from build123d import *

# Parameters (mm, degrees)
BOSS_EXTRUDE1_DEPTH = 100.5


with BuildPart() as part:
    # Sketch1 → Boss-Extrude1 (new body)
    with BuildSketch(Plane(origin=(0, 0, 0), x_dir=(0, 0, -1), z_dir=(1, 0, 0))):
        with BuildLine():
            Line((-15, 13), (-15, 4))
            Line((-15, 4), (-13, 4))
            Line((-13, 4), (-13, 8.25))
            Line((-13, 8.25), (-9.664213562, 8.25))
            Line((-9.664213562, 8.25), (-6, 4.585786438))
            Line((-6, 4.585786438), (-6, -4.585786438))
            Line((-6, -4.585786438), (-9.664213562, -8.25))
            Line((-9.664213562, -8.25), (-13, -8.25))
            Line((-13, -8.25), (-13, -4))
            Line((-13, -4), (-15, -4))
            Line((-15, -4), (-15, -13))
            ThreePointArc((-15, -13), (-14.414213562, -14.414213562), (-13, -15))
            Line((-13, -15), (-4, -15))
            Line((-4, -15), (-4, -13))
            Line((-4, -13), (-8.25, -13))
            Line((-8.25, -13), (-8.25, -9.664213562))
            Line((-8.25, -9.664213562), (-4.585786438, -6))
            Line((-4.585786438, -6), (4.585786438, -6))
            Line((4.585786438, -6), (8.25, -9.664213562))
            Line((8.25, -9.664213562), (8.25, -13))
            Line((8.25, -13), (4, -13))
            Line((4, -13), (4, -15))
            Line((4, -15), (13, -15))
            ThreePointArc((13, -15), (14.414213562, -14.414213562), (15, -13))
            Line((15, -13), (15, -4))
            Line((15, -4), (13, -4))
            Line((13, -4), (13, -8.25))
            Line((13, -8.25), (9.664213562, -8.25))
            Line((9.664213562, -8.25), (6, -4.585786438))
            Line((6, -4.585786438), (6, 4.585786438))
            Line((6, 4.585786438), (9.664213562, 8.25))
            Line((9.664213562, 8.25), (13, 8.25))
            Line((13, 8.25), (13, 4))
            Line((13, 4), (15, 4))
            Line((15, 4), (15, 13))
            ThreePointArc((15, 13), (14.414213562, 14.414213562), (13, 15))
            Line((13, 15), (4, 15))
            Line((4, 15), (4, 13))
            Line((4, 13), (8.25, 13))
            Line((8.25, 13), (8.25, 9.664213562))
            Line((8.25, 9.664213562), (4.585786438, 6))
            Line((4.585786438, 6), (-4.585786438, 6))
            Line((-4.585786438, 6), (-8.25, 9.664213562))
            Line((-8.25, 9.664213562), (-8.25, 13))
            Line((-8.25, 13), (-4, 13))
            Line((-4, 13), (-4, 15))
            Line((-4, 15), (-13, 15))
            ThreePointArc((-13, 15), (-14.414213562, 14.414213562), (-15, 13))
        make_face()
        with BuildLine():
            Line((-9.539070071, 11.338915743), (-9.918883282, 12.361530981))
            ThreePointArc((-9.918883282, 12.361530981), (-13.043502884, 13.043502884), (-12.361530981, 9.918883282))
            Line((-12.361530981, 9.918883282), (-11.338915743, 9.539070071))
            ThreePointArc((-11.338915743, 9.539070071), (-9.861522369, 9.861522369), (-9.539070071, 11.338915743))
        make_face(mode=Mode.SUBTRACT)
        with BuildLine():
            Line((9.918883282, 12.361530981), (9.539070071, 11.338915743))
            ThreePointArc((9.539070071, 11.338915743), (9.861522369, 9.861522369), (11.338915743, 9.539070071))
            Line((11.338915743, 9.539070071), (12.361530981, 9.918883282))
            ThreePointArc((12.361530981, 9.918883282), (13.043502884, 13.043502884), (9.918883282, 12.361530981))
        make_face(mode=Mode.SUBTRACT)
        with BuildLine():
            Line((12.361530981, -9.918883282), (11.338915743, -9.539070071))
            ThreePointArc((11.338915743, -9.539070071), (9.861522369, -9.861522369), (9.539070071, -11.338915743))
            Line((9.539070071, -11.338915743), (9.918883282, -12.361530981))
            ThreePointArc((9.918883282, -12.361530981), (13.043502884, -13.043502884), (12.361530981, -9.918883282))
        make_face(mode=Mode.SUBTRACT)
        with BuildLine():
            Line((-11.338915743, -9.539070071), (-12.361530981, -9.918883282))
            ThreePointArc((-12.361530981, -9.918883282), (-13.043502884, -13.043502884), (-9.918883282, -12.361530981))
            Line((-9.918883282, -12.361530981), (-9.539070071, -11.338915743))
            ThreePointArc((-9.539070071, -11.338915743), (-9.861522369, -9.861522369), (-11.338915743, -9.539070071))
        make_face(mode=Mode.SUBTRACT)
        with BuildLine():
            Line((-4.8, -2.644433572), (-4.8, -4.5))
            ThreePointArc((-4.8, -4.5), (-4.712132034, -4.712132034), (-4.5, -4.8))
            Line((-4.5, -4.8), (-2.644433572, -4.8))
            ThreePointArc((-2.644433572, -4.8), (-2.615679847, -4.79861886), (-2.587190874, -4.794488155))
            Line((-2.587190874, -4.794488155), (-1.742757301, -4.630346896))
            ThreePointArc((-1.742757301, -4.630346896), (-1.568512625, -4.526682207), (-1.5, -4.335858741))
            Line((-1.5, -4.335858741), (-1.5, -3.5))
            ThreePointArc((-1.5, -3.5), (-1.374371458, -3.255879959), (-1.102702703, -3.216216216))
            ThreePointArc((-1.102702703, -3.216216216), (0, -3.4), (1.102702703, -3.216216216))
            ThreePointArc((1.102702703, -3.216216216), (1.374371458, -3.255879959), (1.5, -3.5))
            Line((1.5, -3.5), (1.5, -4.335858741))
            ThreePointArc((1.5, -4.335858741), (1.568512625, -4.526682207), (1.742757301, -4.630346896))
            Line((1.742757301, -4.630346896), (2.587190874, -4.794488155))
            ThreePointArc((2.587190874, -4.794488155), (2.615679847, -4.79861886), (2.644433572, -4.8))
            Line((2.644433572, -4.8), (4.5, -4.8))
            ThreePointArc((4.5, -4.8), (4.712132034, -4.712132034), (4.8, -4.5))
            Line((4.8, -4.5), (4.8, -2.644433572))
            ThreePointArc((4.8, -2.644433572), (4.79861886, -2.615679847), (4.794488155, -2.587190874))
            Line((4.794488155, -2.587190874), (4.630346896, -1.742757301))
            ThreePointArc((4.630346896, -1.742757301), (4.526682207, -1.568512625), (4.335858741, -1.5))
            Line((4.335858741, -1.5), (3.5, -1.5))
            ThreePointArc((3.5, -1.5), (3.255879959, -1.374371458), (3.216216216, -1.102702703))
            ThreePointArc((3.216216216, -1.102702703), (3.4, 0), (3.216216216, 1.102702703))
            ThreePointArc((3.216216216, 1.102702703), (3.255879959, 1.374371458), (3.5, 1.5))
            Line((3.5, 1.5), (4.335858741, 1.5))
            ThreePointArc((4.335858741, 1.5), (4.526682207, 1.568512625), (4.630346896, 1.742757301))
            Line((4.630346896, 1.742757301), (4.794488155, 2.587190874))
            ThreePointArc((4.794488155, 2.587190874), (4.79861886, 2.615679847), (4.8, 2.644433572))
            Line((4.8, 2.644433572), (4.8, 4.5))
            ThreePointArc((4.8, 4.5), (4.712132034, 4.712132034), (4.5, 4.8))
            Line((4.5, 4.8), (2.644433572, 4.8))
            ThreePointArc((2.644433572, 4.8), (2.615679847, 4.79861886), (2.587190874, 4.794488155))
            Line((2.587190874, 4.794488155), (1.742757301, 4.630346896))
            ThreePointArc((1.742757301, 4.630346896), (1.568512625, 4.526682207), (1.5, 4.335858741))
            Line((1.5, 4.335858741), (1.5, 3.5))
            ThreePointArc((1.5, 3.5), (1.374371458, 3.255879959), (1.102702703, 3.216216216))
            ThreePointArc((1.102702703, 3.216216216), (0, 3.4), (-1.102702703, 3.216216216))
            ThreePointArc((-1.102702703, 3.216216216), (-1.374371458, 3.255879959), (-1.5, 3.5))
            Line((-1.5, 3.5), (-1.5, 4.335858741))
            ThreePointArc((-1.5, 4.335858741), (-1.568512625, 4.526682207), (-1.742757301, 4.630346896))
            Line((-1.742757301, 4.630346896), (-2.587190874, 4.794488155))
            ThreePointArc((-2.587190874, 4.794488155), (-2.615679847, 4.79861886), (-2.644433572, 4.8))
            Line((-2.644433572, 4.8), (-4.5, 4.8))
            ThreePointArc((-4.5, 4.8), (-4.712132034, 4.712132034), (-4.8, 4.5))
            Line((-4.8, 4.5), (-4.8, 2.644433572))
            ThreePointArc((-4.8, 2.644433572), (-4.79861886, 2.615679847), (-4.794488155, 2.587190874))
            Line((-4.794488155, 2.587190874), (-4.630346896, 1.742757301))
            ThreePointArc((-4.630346896, 1.742757301), (-4.526682207, 1.568512625), (-4.335858741, 1.5))
            Line((-4.335858741, 1.5), (-3.5, 1.5))
            ThreePointArc((-3.5, 1.5), (-3.255879959, 1.374371458), (-3.216216216, 1.102702703))
            ThreePointArc((-3.216216216, 1.102702703), (-3.4, 0), (-3.216216216, -1.102702703))
            ThreePointArc((-3.216216216, -1.102702703), (-3.255879959, -1.374371458), (-3.5, -1.5))
            Line((-3.5, -1.5), (-4.335858741, -1.5))
            ThreePointArc((-4.335858741, -1.5), (-4.526682207, -1.568512625), (-4.630346896, -1.742757301))
            Line((-4.630346896, -1.742757301), (-4.794488155, -2.587190874))
            ThreePointArc((-4.794488155, -2.587190874), (-4.79861886, -2.615679847), (-4.8, -2.644433572))
        make_face(mode=Mode.SUBTRACT)
    extrude(amount=BOSS_EXTRUDE1_DEPTH)


solid = part.part
Source: CAD feature listing. Evaluate the final solid. Frame: model axes, mm. A direction names the side the tool comes from. Give positions to 0.01 mm unless a question says otherwise; leave off trailing zeros. Write item = value, one per line.
Q1. First-contact query: pin 1 (0.6 mm diameter, centred on x = 74.5, y = 14.5, fed in from -Z); pin 2 (2 mm diameter, centred on y = 7, z = 6, fed in from -X). Flat tips, straight axial feed; report the tip coordinate or a pass-through.
Here are the results:
pin_1 = -14.6
pin_2 = 0
Q2. Cut plane A-A on x = 23. State how many separate pieces and enclosed holes the cut face has, then the cut area to 3 significant figures.
Here are the results:
separate_pieces = 1
enclosed_holes = 5
area = 299 mm²
Q3. Reachability of faces 4 (the face through (50, 6, -13)), 5 (the face through (50, 14, -4)), 6 (the face through (50, 8, -15)) from +Z, -Z, +X, -X, +Y, -Y: full face, straight path, thin tool, end or side. Return the list, or none.
Here are the results:
face_4 = +X, -X
face_5 = +X, -X, +Y
face_6 = -Z, +X, -X, +Y, -Y
Q4. Line query: line 1 (Y direction, x = 50.5, z = -11.7); line 2 (Z direction, x = 19, y = 12.75). Output: solid intervals per line, ascending. Write a range as from..to.
Here are the results:
line_1 = -15..-13.6, -9.67..-8.25, 8.25..9.67, 13.6..15
line_2 = -15..-13.28, -10.12..-8.25, 8.25..10.12, 13.28..15
Q5. Mould query, pull axis Z, two halves, no side actions, for faces 1 (the face through (50, 15, 8)), 2 (the face through (50, -9, -15)), 3 (the face through (49.546, -9.877, 9.846)). Classes: +Z half, -Z half, draft (parallel to the pull), parting line (faces both ways), or undercut.
Here are the results:
face_1 = draft
face_2 = -Z half
face_3 = undercut
